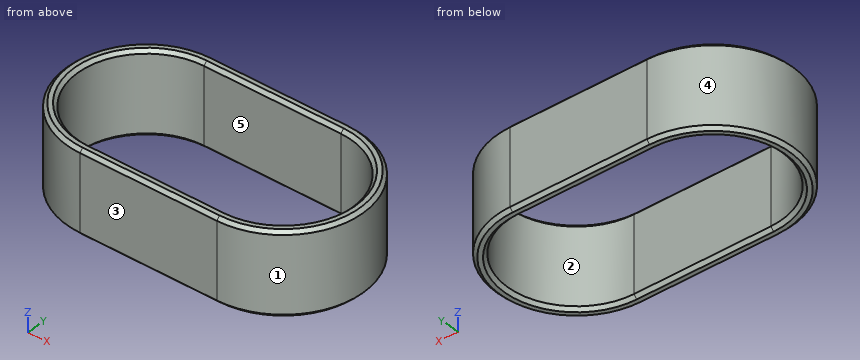
from build123d import *

# Parameters (mm, degrees)
PAD_DEPTH    = 15
CHAMFER_SIZE = 0.6


with BuildPart() as part:
    # Sketch002 → Pad (new body)
    with BuildSketch(Plane.XY):
        with BuildLine():
            ThreePointArc((-12.5, 14.5), (-27, 0), (-12.5, -14.5))
            Line((-12.5, -14.5), (12.5, -14.5))
            ThreePointArc((12.5, -14.5), (27, 0), (12.5, 14.5))
            Line((-12.5, 14.5), (12.5, 14.5))
        make_face()
        with BuildLine():
            ThreePointArc((-12.5, 12.5), (-25, 0), (-12.5, -12.5))
            Line((-12.5, -12.5), (12.5, -12.5))
            ThreePointArc((12.5, -12.5), (25, 0), (12.5, 12.5))
            Line((-12.5, 12.5), (12.5, 12.5))
        make_face(mode=Mode.SUBTRACT)
    extrude(amount=PAD_DEPTH)

    # Chamfer
    chamfer_edges = [part.edges().sort_by_distance(p)[0] for p in [
        (-27, 0, 15),
        (0, -14.5, 15),
        (27, 0, 15),
        (0, 14.5, 15),
        (-25, 0, 15),
        (0, -12.5, 15),
        (25, 0, 15),
        (0, 12.5, 15),
        (-27, 0, 0),
        (0, -14.5, 0),
        (27, 0, 0),
        (0, 14.5, 0),
        (-25, 0, 0),
        (0, -12.5, 0),
        (25, 0, 0),
        (0, 12.5, 0),
    ]]
    chamfer(chamfer_edges, length=CHAMFER_SIZE)


solid = part.part
Geometry: final body of the model. Coordinates: model frame, mm. Face numbers are marked on the shaded views. A direction names the side the tool comes from. Round coordinates to 2 decimals unless told otherwise and drop trailing zeros. Loops run counter-clockwise (first coordinate to the right, second up) from the corner with the lowest first, then second, coordinate; pieces in that order, holes last. Notation, with made-up numbers: M -8,10 L 40,10 A34 cw 40,40 Z; hole C -28.5,31.5 d4. An arc over 180 degrees is marked long. Put each result on its own line as item: value. Start each with the question number.
(1) Draft query along X for the marked faces 3, 4 and 5. Return one class per face: +X half, -X half, draft (parallel to the pull), parting line (faces both ways), or undercut.
(2) Section query B-B (x = -2). Return loops of the section in (y, z), then the cut area to 3 significant figures.
(3) Set-up query: the marked faces 1 and 2. Return all of +Z, -Z, +X, -X, +Y, -Y with unobstructed straight access to the full face (end or side cutting, diameter ignored); none if empty.
(4) Section query A-A (y = 0). Return loops of the section in (x, z).
(5) Section query C-C (z = 4.75). Return loops of the section in (x, y), then the cut area to 3 significant figures.
(6) Contact query for flat-ended pins moving along their axis: pin 1 Ø8 at (x, z) = (17, 3.5) entering from +Y; pin 2 Ø4 at (y, z) = (-3.5, 7) entering from -X; pin 3 Ø6 at (x, z) = (21, 2) entering from +Y; pin 4 Ø5 at (x, z) = (14, 13) entering from -Y. Output: stop coordinate, or through.
(7) Material intervals for line 1 along Y through (x, z) = (-8, 4); line 2 along X through (y, z) = (0.5, 4); line 3 along Y through (x, z) = (-22, 8.75), sorted ascending. Write a range as [from, to].
Findings below:
1. face 3: draft
1. face 4: -X half
1. face 5: undercut
2. outline: M -14.5,0.6 L -13.9,0 L -13.1,0 L -12.5,0.6 L -12.5,14.4 L -13.1,15 L -13.9,15 L -14.5,14.4 Z; M 12.5,0.6 L 13.1,0 L 13.9,0 L 14.5,0.6 L 14.5,14.4 L 13.9,15 L 13.1,15 L 12.5,14.4 Z
2. area: 58.6 mm2
3. face 1: +Z, -Z, +X
3. face 2: +Z, -Z
4. outline: M -27,0.6 L -26.4,0 L -25.6,0 L -25,0.6 L -25,14.4 L -25.6,15 L -26.4,15 L -27,14.4 Z; M 25,0.6 L 25.6,0 L 26.4,0 L 27,0.6 L 27,14.4 L 26.4,15 L 25.6,15 L 25,14.4 Z
5. outline: M -12.5,-14.5 L 12.5,-14.5 A14.5 ccw 12.5,14.5 L -12.5,14.5 A14.5 ccw Z; hole M -12.5,-12.5 L 12.5,-12.5 A12.5 ccw 12.5,12.5 L -12.5,12.5 A12.5 ccw Z
5. area: 270 mm2
6. pin 1: stops at y = 14.49
6. pin 2: stops at x = -26.92
6. pin 3: stops at y = 13.42
6. pin 4: stops at y = -14.5
7. line 1: y = [-14.5, -12.5], [12.5, 14.5]
7. line 2: x = [-26.99, -24.99], [24.99, 26.99]
7. line 3: y = [-10.95, -8.12], [8.12, 10.95]
